```python
from build123d import *
from OCP.BRepFilletAPI import BRepFilletAPI_MakeChamfer

# Parameters (mm, degrees)
SKETCH1_R                                           = 11
BOSS_EXTRUDE1_DEPTH                                 = 18
CUT_EXTRUDE4_DEPTH                                  = 60
CUT_EXTRUDE5_DEPTH                                  = 10
CHAMFER1_SIZE                                       = 3.639702343
CHAMFER1_SIZE_2                                     = 10
CUT_EXTRUDE6_DEPTH                                  = 42.9
CUT_EXTRUDE7_START                                  = -11.1
CUT_EXTRUDE7_DEPTH                                  = 11.1
CBORE_FOR_M3_HEX_SOCKET_HEAD_CAP_SCREW2_D           = 3.4
CBORE_FOR_M3_HEX_SOCKET_HEAD_CAP_SCREW2_DEPTH       = 8
CBORE_FOR_M3_HEX_SOCKET_HEAD_CAP_SCREW2_CBORE_D     = 6.5
CBORE_FOR_M3_HEX_SOCKET_HEAD_CAP_SCREW2_CBORE_DEPTH = 3.4
CBORE_FOR_M3_HEX_SOCKET_HEAD_CAP_SCREW2_TIP         = 1.021463052
CBORE_FOR_M4_HEX_SOCKET_HEAD_CAP_SCREW1_D           = 4.5
CBORE_FOR_M4_HEX_SOCKET_HEAD_CAP_SCREW1_DEPTH       = 8
CBORE_FOR_M4_HEX_SOCKET_HEAD_CAP_SCREW1_CBORE_D     = 8
CBORE_FOR_M4_HEX_SOCKET_HEAD_CAP_SCREW1_CBORE_DEPTH = 4.4
CBORE_FOR_M4_HEX_SOCKET_HEAD_CAP_SCREW1_TIP         = 1.351936393
CBORE_FOR_M4_HEX_SOCKET_HEAD_CAP_SCREW2_D           = 4.5
CBORE_FOR_M4_HEX_SOCKET_HEAD_CAP_SCREW2_DEPTH       = 8
CBORE_FOR_M4_HEX_SOCKET_HEAD_CAP_SCREW2_CBORE_D     = 8
CBORE_FOR_M4_HEX_SOCKET_HEAD_CAP_SCREW2_CBORE_DEPTH = 4.4
CBORE_FOR_M4_HEX_SOCKET_HEAD_CAP_SCREW2_TIP         = 1.351936393
M4_CLEARANCE_HOLE1_D                                = 4.5
M4_CLEARANCE_HOLE1_DEPTH                            = 8
M4_CLEARANCE_HOLE1_TIP                              = 1.351936393
F_4_0MM_DOWEL_HOLE1_D                               = 4
F_4_0MM_DOWEL_HOLE1_DEPTH                           = 8
F_4_0MM_DOWEL_HOLE1_TIP                             = 1.201721238


with BuildPart() as part:
    # Sketch1 → Boss-Extrude1 (new body)
    with BuildSketch(Plane.XY):
        Polygon((39.1, 65), (39.1, 45), (19.1, 45), (19.1, 65), (11.1, 65), (0, 31), (0, 0), (90, 0), (90, 5), (72.831044759, 45), (47.1, 65), align=None)
        with Locations((40, 22.15)):
            Circle(SKETCH1_R, mode=Mode.SUBTRACT)
    extrude(amount=BOSS_EXTRUDE1_DEPTH)

    # Sketch5 → Cut-Extrude4 (cut)
    with BuildSketch(Plane(origin=(0, 65, 0), x_dir=(1, 0, 0), z_dir=(0, 1, 0))):
        with BuildLine():
            Line((90, -15), (80, -15))
            ThreePointArc((80, -15), (74, -9), (80, -3))
            Line((80, -3), (90, -3))
            ThreePointArc((90, -3), (96, -9), (90, -15))
        make_face()
    extrude(amount=-CUT_EXTRUDE4_DEPTH, mode=Mode.SUBTRACT)

    # Sketch6 → Cut-Extrude5 (cut)
    with BuildSketch(Plane.XY.offset(18)):
        Polygon((19.1, 45), (15, 32.441441441), (15, 0), (65, 0), (65, 28.75503195), (44.1, 45), align=None)
    extrude(amount=-CUT_EXTRUDE5_DEPTH, mode=Mode.SUBTRACT)

    # Chamfer1
    chamfer1_edges_1 = [part.edges().sort_by_distance(p)[0] for p in [
        (15, 16.220720721, 18),
    ]]
    chamfer1_side_1 = [part.faces().sort_by_distance(p)[0] for p in [
        (14.927205953, 16.220720721, 18),
    ]]
    chamfer1_edges_2 = [part.edges().sort_by_distance(p)[0] for p in [
        (65, 14.377515975, 18),
    ]]
    chamfer1_side_2 = [part.faces().sort_by_distance(p)[0] for p in [
        (65.072794047, 14.377515975, 18),
    ]]
    chamfer1 = BRepFilletAPI_MakeChamfer(part.part.solid().wrapped)
    for e in chamfer1_edges_1:
        chamfer1.Add(CHAMFER1_SIZE - 0.0001, CHAMFER1_SIZE_2 - 0.0001, e.wrapped, chamfer1_side_1[0].wrapped)
    for e in chamfer1_edges_2:
        chamfer1.Add(CHAMFER1_SIZE - 0.0001, CHAMFER1_SIZE_2 - 0.0001, e.wrapped, chamfer1_side_2[0].wrapped)
    add(Compound.cast(chamfer1.Shape()), mode=Mode.REPLACE)  # a hair under: the kernel refuses the full size

    # Sketch7 → Cut-Extrude6 (cut)
    with BuildSketch(Plane(origin=(90, 0, 0), x_dir=(0, 0, -1), z_dir=(1, 0, 0))):
        with BuildLine():
            Line((-3, 65), (-3, 55))
            ThreePointArc((-3, 55), (-9, 49), (-15, 55))
            Line((-15, 55), (-15, 65))
            ThreePointArc((-15, 65), (-9, 71), (-3, 65))
        make_face()
    extrude(amount=-CUT_EXTRUDE6_DEPTH, mode=Mode.SUBTRACT)

    # Sketch8 → Cut-Extrude7 (cut)
    with BuildSketch(Plane.ZY.offset(CUT_EXTRUDE7_START)):
        with BuildLine():
            Line((15, 65), (15, 55))
            ThreePointArc((15, 55), (9, 49), (3, 55))
            Line((3, 55), (3, 65))
            ThreePointArc((3, 65), (9, 71), (15, 65))
        make_face()
    extrude(amount=CUT_EXTRUDE7_DEPTH, mode=Mode.SUBTRACT)

    # CBORE for M3 Hex Socket Head Cap Screw2
    with Locations(Plane.XY.offset(8)):
        with Locations((40, 37.15), (52.990381057, 14.65), (27.009618943, 14.65)):
            CounterBoreHole(CBORE_FOR_M3_HEX_SOCKET_HEAD_CAP_SCREW2_D / 2, CBORE_FOR_M3_HEX_SOCKET_HEAD_CAP_SCREW2_CBORE_D / 2, CBORE_FOR_M3_HEX_SOCKET_HEAD_CAP_SCREW2_CBORE_DEPTH, depth=CBORE_FOR_M3_HEX_SOCKET_HEAD_CAP_SCREW2_DEPTH)
            with Locations((0, 0, -(CBORE_FOR_M3_HEX_SOCKET_HEAD_CAP_SCREW2_DEPTH + CBORE_FOR_M3_HEX_SOCKET_HEAD_CAP_SCREW2_TIP / 2))):  # 118° drill point
                Cone(0, CBORE_FOR_M3_HEX_SOCKET_HEAD_CAP_SCREW2_D / 2, CBORE_FOR_M3_HEX_SOCKET_HEAD_CAP_SCREW2_TIP, mode=Mode.SUBTRACT)

    # CBORE for M4 Hex Socket Head Cap Screw1
    with Locations(Plane(origin=(47.1, 0, 0), x_dir=(0, 0, -1), z_dir=(1, 0, 0))):
        with Locations((-9, 55)):
            CounterBoreHole(CBORE_FOR_M4_HEX_SOCKET_HEAD_CAP_SCREW1_D / 2, CBORE_FOR_M4_HEX_SOCKET_HEAD_CAP_SCREW1_CBORE_D / 2, CBORE_FOR_M4_HEX_SOCKET_HEAD_CAP_SCREW1_CBORE_DEPTH, depth=CBORE_FOR_M4_HEX_SOCKET_HEAD_CAP_SCREW1_DEPTH)
            with Locations((0, 0, -(CBORE_FOR_M4_HEX_SOCKET_HEAD_CAP_SCREW1_DEPTH + CBORE_FOR_M4_HEX_SOCKET_HEAD_CAP_SCREW1_TIP / 2))):  # 118° drill point
                Cone(0, CBORE_FOR_M4_HEX_SOCKET_HEAD_CAP_SCREW1_D / 2, CBORE_FOR_M4_HEX_SOCKET_HEAD_CAP_SCREW1_TIP, mode=Mode.SUBTRACT)

    # CBORE for M4 Hex Socket Head Cap Screw2
    with Locations(Plane.ZY.offset(-11.1)):
        with Locations((9, 55)):
            CounterBoreHole(CBORE_FOR_M4_HEX_SOCKET_HEAD_CAP_SCREW2_D / 2, CBORE_FOR_M4_HEX_SOCKET_HEAD_CAP_SCREW2_CBORE_D / 2, CBORE_FOR_M4_HEX_SOCKET_HEAD_CAP_SCREW2_CBORE_DEPTH, depth=CBORE_FOR_M4_HEX_SOCKET_HEAD_CAP_SCREW2_DEPTH)
            with Locations((0, 0, -(CBORE_FOR_M4_HEX_SOCKET_HEAD_CAP_SCREW2_DEPTH + CBORE_FOR_M4_HEX_SOCKET_HEAD_CAP_SCREW2_TIP / 2))):  # 118° drill point
                Cone(0, CBORE_FOR_M4_HEX_SOCKET_HEAD_CAP_SCREW2_D / 2, CBORE_FOR_M4_HEX_SOCKET_HEAD_CAP_SCREW2_TIP, mode=Mode.SUBTRACT)

    # M4 Clearance Hole1
    with Locations(Plane(origin=(0, 5, 0), x_dir=(1, 0, 0), z_dir=(0, 1, 0))):
        with Locations((80, -9)):
            Hole(M4_CLEARANCE_HOLE1_D / 2, depth=M4_CLEARANCE_HOLE1_DEPTH)
            with Locations((0, 0, -(M4_CLEARANCE_HOLE1_DEPTH + M4_CLEARANCE_HOLE1_TIP / 2))):  # 118° drill point
                Cone(0, M4_CLEARANCE_HOLE1_D / 2, M4_CLEARANCE_HOLE1_TIP, mode=Mode.SUBTRACT)

    # Ø4.0mm Dowel Hole1
    with Locations(Plane(origin=(0, 0, 0), x_dir=(-1, 0, 0), z_dir=(0, -1, 0))):
        with Locations((-7, -12), (-7, -6)):
            Hole(F_4_0MM_DOWEL_HOLE1_D / 2, depth=F_4_0MM_DOWEL_HOLE1_DEPTH)
            with Locations((0, 0, -(F_4_0MM_DOWEL_HOLE1_DEPTH + F_4_0MM_DOWEL_HOLE1_TIP / 2))):  # 118° drill point
                Cone(0, F_4_0MM_DOWEL_HOLE1_D / 2, F_4_0MM_DOWEL_HOLE1_TIP, mode=Mode.SUBTRACT)


solid = part.part
```
Source: CAD feature listing. Evaluate the final solid. Frame: model axes, mm. A direction names the side the tool comes from. Round coordinates to 2 decimals unless told otherwise and drop trailing zeros. Loops run counter-clockwise (first coordinate to the right, second up) from the corner with the lowest first, then second, coordinate; pieces in that order, holes last.
1. Access query for faces 4 (the flat face through (19.1, 52.6, 8.9)), 5 (the flat face through (10, 59, 3)), 6 (the flat face through (13.206, 12.843, 12.93)), 7 (the flat face through (83, 12, 15)), 8 (the cylindrical face through (17.33, 57.23, 9.29)). Directions: +Z, -Z, +X, -X, +Y, -Y. A direction counts if a zero-diameter tool reaches every point of the face in a straight line with its end or side. Return the directions, or none.
2. Mould query, pull axis Y, two halves, no side actions, for faces 1 (the cylindrical face through (28.509, 11.767, 6.324)), 2 (the flat face through (16.144, 35.947, 13.07)), 3 (the flat face through (9, 33, 18)). Classes: released by +Y, released by -Y, zero draft, split by the parting line, or undercut.
3. Ray query, L1, parallel to Z at x = 7, y = 2.75; L2, parallel to Y at x = 40, z = 2.2; L3, parallel to Z at x = 52.5, y = 60. Return the intervals inside material, ascending.
4. Section query C-C on z = 9. Give the number of separate pieces and of enclosed holes in the cut face, and give its area (3 significant figures).
5. Contact query for flat-ended pins moving along their axis: pin 1 (4 mm diameter, centred on y = 46.5, z = 6, fed in from -X); pin 2 (3 mm diameter, centred on x = 60, z = 13, fed in from +Y); pin 3 (6 mm diameter, centred on x = 44.5, y = 28.5, fed in from -Z); pin 4 (2 mm diameter, centred on x = 57.5, z = 8, fed in from +Y). Output: stop coordinate, or through.
6. Section query A-A on x = 40. Output: boundary loops of the cut face in (y, z).
Answers below:
1. face 4: +Z, -Z, +Y
1. face 5: -X, +Y
1. face 6: +Z, -Y
1. face 7: +X, +Y
1. face 8: +X, -X
2. face 1: undercut
2. face 2: released by -Y
2. face 3: zero draft
3. L1: z = 0 to 4, 8 to 10, 14 to 18
3. L2: y = 0 to 11.15, 33.15 to 35.45, 38.85 to 65
3. L3: z = 0 to 3, 15 to 18
4. separate pieces: 5
4. enclosed holes: 0
4. area: 1,610 mm2
5. pin 1: stops at x = 4.41
5. pin 2: stops at y = 52.6
5. pin 3: passes through
5. pin 4: stops at y = 49.34
6. outline: (0, 0) - (11.15, 0) - (11.15, 8) - (0, 8) - close; (33.15, 0) - (35.45, 0) - (35.45, 4.6) - (33.9, 4.6) - (33.9, 8) - (33.15, 8) - close; (38.85, 0) - (65, 0) - (65, 18) - (45, 18) - (45, 8) - (40.4, 8) - (40.4, 4.6) - (38.85, 4.6) - close; hole circle Ø4.5 at (55, 9)
